Can you work these out from the model? Positions are in its coordinate system, mm. Face numbers are marked on the shaded views. A direction names the side the tool comes from. Give positions to 0.01 mm unless a question says otherwise; leave off trailing zeros. Write each loop counter-clockwise with the first axis right and the second up, starting at its lowest first coordinate (ties: lowest second). Pieces come first, ordered by that corner, then holes.
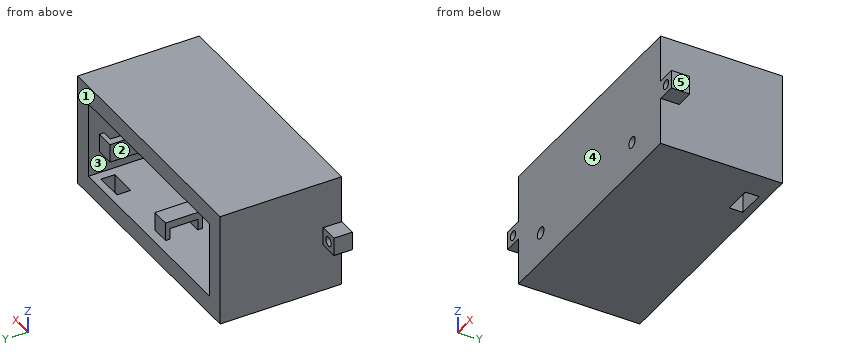
from build123d import *

# Parameters (mm, degrees)
SKETCH1_W                 = 85.09
SKETCH1_H                 = 39.00542054
SKETCH1_W_2               = 72.39
SKETCH1_H_2               = 26.30542054
BOSS_EXTRUDE1_DEPTH       = 35.56
SKETCH1_3_W               = 85.09
SKETCH1_3_H               = 39.00542054
SKETCH1_3_R               = 1.967283446
SKETCH1_3_W_2             = 3.175
SKETCH1_3_H_2             = 3.175
SKETCH1_3_R_2             = 1.397
BOSS_EXTRUDE2_DEPTH       = 6.35
SKETCH1_4_W               = 6.35
SKETCH1_4_H               = 6.35
SKETCH1_4_R               = 1.5875
BOSS_EXTRUDE3_DEPTH       = 6.35
SKETCH1_5_R               = 1.967283446
BOSS_EXTRUDE4_DEPTH       = 2.54
SKETCH2_W                 = 6.35
SKETCH2_H                 = 1.5875
SKETCH2_H_2               = 9.525
BOSS_EXTRUDE8_DEPTH       = 6.35
SKETCH2_4_W               = 6.35
SKETCH2_4_H               = 9.525
CUT_EXTRUDE1_DEPTH        = 3.81
SKETCH1_10_R              = 1.905
SKETCH1_10_R_2            = 1.397
SKETCH1_10_R_3            = 1.967283446
CUT_EXTRUDE4_DEPTH        = 98.832500687
SKETCH1_11_W              = 3.175
SKETCH1_11_H              = 3.175
BOSS_EXTRUDE11_DEPTH      = 2.54
BOSS_EXTRUDE11_DEPTH_BACK = 6.35
SKETCH6_W                 = 6.35
SKETCH6_H                 = 9.525
SKETCH6_H_2               = 1.5875
BOSS_EXTRUDE12_DEPTH      = 6.35
SKETCH6_8_W               = 6.35
SKETCH6_8_H               = 9.525
CUT_EXTRUDE5_DEPTH        = 3.81
SKETCH8_W                 = 9.525
SKETCH8_H                 = 4.7625
CUT_EXTRUDE6_DEPTH        = 18.542


with BuildPart() as part:
    # Sketch1 → Boss-Extrude1 (new body)
    with BuildSketch(Plane(origin=(0, 0, 0), x_dir=(1, 0, 0), z_dir=(0, 1, 0))):
        with Locations((36.195, 13.15271027)):
            Rectangle(SKETCH1_W, SKETCH1_H)
        with Locations((36.195, 13.15271027)):
            Rectangle(SKETCH1_W_2, SKETCH1_H_2, mode=Mode.SUBTRACT)
    extrude(amount=BOSS_EXTRUDE1_DEPTH)

    # Sketch1_3 → Boss-Extrude2 (add)
    with BuildSketch(Plane(origin=(0, 0, 0), x_dir=(1, 0, 0), z_dir=(0, 1, 0))):
        with Locations((36.195, 13.15271027)):
            Rectangle(SKETCH1_3_W, SKETCH1_3_H)
        with Locations(Location((6.985, 22.098, 0), (0, 0, 270))):
            Circle(SKETCH1_3_R, mode=Mode.SUBTRACT)
        with Locations((51.59375, 1.997278049)):
            Rectangle(SKETCH1_3_W_2, SKETCH1_3_H_2, mode=Mode.SUBTRACT)
        with Locations(Location((61.595, 21.999778049, 0), (0, 0, 270))):
            Circle(SKETCH1_3_R_2, mode=Mode.SUBTRACT)
    extrude(amount=-BOSS_EXTRUDE2_DEPTH)

    # Sketch1_4 → Boss-Extrude3 (add)
    with BuildSketch(Plane(origin=(0, 0, 0), x_dir=(1, 0, 0), z_dir=(0, 1, 0))):
        with Locations((-9.525, 13.15271027)):
            Rectangle(SKETCH1_4_W, SKETCH1_4_H)
        with Locations(Location((-9.525, 13.15271027, 0), (0, 0, 270))):
            Circle(SKETCH1_4_R, mode=Mode.SUBTRACT)
        with Locations((81.915, 13.15271027)):
            Rectangle(SKETCH1_4_W, SKETCH1_4_H)
        with Locations(Location((81.915, 13.15271027, 0), (0, 0, 270))):
            Circle(SKETCH1_4_R, mode=Mode.SUBTRACT)
    extrude(amount=-BOSS_EXTRUDE3_DEPTH)

    # Sketch1_5 → Boss-Extrude4 (add)
    with BuildSketch(Plane(origin=(0, 0, 0), x_dir=(1, 0, 0), z_dir=(0, 1, 0))):
        with Locations(Location((6.985, 22.098, 0), (0, 0, 270))):
            Circle(SKETCH1_5_R)
    extrude(amount=-BOSS_EXTRUDE4_DEPTH)

    # Sketch2 → Boss-Extrude8 (add)
    with BuildSketch(Plane.XY.offset(-26.30542054)):
        with Locations((34.925, 20.47875)):
            Rectangle(SKETCH2_W, SKETCH2_H)
        with Locations((34.925, 26.035)):
            Rectangle(SKETCH2_W, SKETCH2_H_2)
        with Locations((34.925, 31.59125)):
            Rectangle(SKETCH2_W, SKETCH2_H)
    extrude(amount=BOSS_EXTRUDE8_DEPTH)

    # Sketch2_4 → Cut-Extrude1 (cut)
    with BuildSketch(Plane.XY.offset(-26.30542054)):
        with Locations((34.925, 26.035)):
            Rectangle(SKETCH2_4_W, SKETCH2_4_H)
    extrude(amount=CUT_EXTRUDE1_DEPTH, mode=Mode.SUBTRACT)

    # Sketch1_10 → Cut-Extrude4 (cut, through all)
    with BuildSketch(Plane(origin=(0, 0, 0), x_dir=(1, 0, 0), z_dir=(0, 1, 0))):
        with Locations(Location((61.595, 21.999778049, 0), (0, 0, 270))):
            Circle(SKETCH1_10_R)
        with Locations((61.595, 21.999778049)):
            Circle(SKETCH1_10_R_2, mode=Mode.SUBTRACT)
        with Locations(Location((6.985, 22.098, 0), (0, 0, 270))):
            Circle(SKETCH1_10_R_3)
        with Locations(Location((6.985, 22.098, 0), (0, 0, 270))):
            Circle(SKETCH1_10_R_2, mode=Mode.SUBTRACT)
    extrude(amount=-CUT_EXTRUDE4_DEPTH, mode=Mode.SUBTRACT)


with BuildPart() as cut_extrude4_piece_1:
    # of the separate pieces the step leaves, piece 1, a body of its own (cut_extrude4_pieces)
    add(part.part.solids().sort_by_distance((78.74, -6.35, -32.65542054))[0])

    # Sketch1_11 → Boss-Extrude11 (add, two sides)
    with BuildSketch(Plane(origin=(0, 0, 0), x_dir=(1, 0, 0), z_dir=(0, 1, 0))) as boss_extrude11_sk:
        with Locations((51.59375, 1.997278049)):
            Rectangle(SKETCH1_11_W, SKETCH1_11_H)
    extrude(amount=BOSS_EXTRUDE11_DEPTH)
    extrude(boss_extrude11_sk.sketch, amount=-BOSS_EXTRUDE11_DEPTH_BACK)

    # Sketch6 → Boss-Extrude12 (add)
    with BuildSketch(Plane(origin=(72.39, 0, -72.39), x_dir=(0, 0, 1), z_dir=(-1, 0, 0))):
        with Locations((56.87957946, 25.4)):
            Rectangle(SKETCH6_W, SKETCH6_H)
        with Locations((56.87957946, 30.95625)):
            Rectangle(SKETCH6_W, SKETCH6_H_2)
        with Locations((56.87957946, 19.84375)):
            Rectangle(SKETCH6_W, SKETCH6_H_2)
    extrude(amount=BOSS_EXTRUDE12_DEPTH)

    # Sketch6_8 → Cut-Extrude5 (cut)
    with BuildSketch(Plane(origin=(72.39, 0, -72.39), x_dir=(0, 0, 1), z_dir=(-1, 0, 0))):
        with Locations((56.87957946, 25.4)):
            Rectangle(SKETCH6_8_W, SKETCH6_8_H)
    extrude(amount=CUT_EXTRUDE5_DEPTH, mode=Mode.SUBTRACT)

    # Sketch8 → Cut-Extrude6 (cut)
    with BuildSketch(Plane.XY.offset(-26.30542054)):
        with Locations((64.4525, 30.63875)):
            Rectangle(SKETCH8_W, SKETCH8_H)
    extrude(amount=-CUT_EXTRUDE6_DEPTH, mode=Mode.SUBTRACT)


with BuildPart() as cut_extrude4_piece_2:
    # of the separate pieces the step leaves, piece 2, a body of its own (cut_extrude4_pieces)
    add(part.part.solids().sort_by_distance((6.985, -2.54, -20.701))[0])


solid = cut_extrude4_piece_1.part
(1) If we mould it in two halves opening along X, with no side actions, what happens to the marked faces 3, 4 and 5? For each: +X half, -X half, draft (parallel to the pull), parting line (faces both ways), or undercut.
Returned:
face 3: undercut
face 4: draft
face 5: +X half
(2) For the marked faces 1 and 2, which set-ups out of +Z, -Z, +X, -X, +Y, -Y let a thin tool reach every point of the face, with its end or its side?
Returned:
face 1: +Z, -Z, +X, -X, +Y
face 2: +Y
(3) Will these pins go through, and if not, where does the flat tip stop? P1, Ø1.9, axis at x = 83.5, y = -4.5, coming from the -Z side; P2, Ø5, axis at x = -11, y = -4, coming from the +Z side; P3, Ø1, axis at y = 27.5, z = -8, coming from the +X side.
Returned:
P1: stops at z = -16.33
P2: stops at z = -9.98
P3: stops at x = 78.74
(4) If I drill on L1, parallel to Z at x = 57, y = 29; L2, parallel to X at y = 30, z = -17.5; L3, parallel to Z at x = 67, y = 29, over which ranges is the centre line in solid material (lowest first)?
Returned:
L1: z = -32.66 to -26.31, 0 to 6.35
L2: x = -6.35 to 0, 66.04 to 68.58, 72.39 to 78.74
L3: z = -18.69 to -12.34, 0 to 6.35
(5) Imagine slicing it at A-A, the plane x = 24.5. Write out the boundary of the cut face in (y, z).
Returned:
outline: (-6.35, -32.66) - (35.56, -32.66) - (35.56, -26.31) - (0, -26.31) - (0, 0) - (35.56, 0) - (35.56, 6.35) - (-6.35, 6.35) - close
(6) Imagine slicing it at D-D, the plane y = -2.5. Give the number of separate pieces and of enclosed holes in the cut face, plus the area to 3 significant figures.
Returned:
separate pieces: 1
enclosed holes: 4
area: 3,360 mm2
(7) Imagine slicing it at C-C, the plane z = -5. Write out the boundary of the cut face in (x, y), plus the area to 3 significant figures.
Returned:
outline: (-6.35, -6.35) - (78.74, -6.35) - (78.74, 35.56) - (72.39, 35.56) - (72.39, 0) - (0, 0) - (0, 35.56) - (-6.35, 35.56) - close
area: 992 mm2
(8) Imagine slicing it at B-B, the plane y = 9. Write out the boundary of the cut face in (x, z), plus the area to 3 significant figures.
Returned:
outline: (-6.35, -32.66) - (78.74, -32.66) - (78.74, 6.35) - (-6.35, 6.35) - close; hole (0, -26.31) - (72.39, -26.31) - (72.39, 0) - (0, 0) - close
area: 1,410 mm2
